Autodesk Inventor part; units mm, degrees
ref_plane "YZ Plane" through (0, 0, 0) normal (1, 0, 0) x (0, 1, 0)
ref_plane "XZ Plane" through (0, 0, 0) normal (0, 1, 0) x (-1, 0, 0)
ref_plane "XY Plane" through (0, 0, 0) normal (0, 0, 1) x (1, 0, 0)
sketch "Sketch1" plane through (0, 0, 0) normal (0, 1, 0) x (-1, 0, 0)
  circle A0 centre (16.272, 0) radius 2.1
  line L0 (14.741, 3.5) -> (19.6914, 3.5)
  line L1 (14.741, -3.5) -> (19.6914, -3.5)
  line L2 (14.741, 3.5) -> (12, 3.5)
  line L3 (14.741, -3.5) -> (12, -3.5)
  line L4 (-2.9689, 12.1423) -> (-6.8146, 18.8032)
  line L5 (-12.8768, 15.3032) -> (-9.0311, 8.6423)
  line L6 (12, -3.5) -> (19.6914, -3.5)
  line L7 (12, 3.5) -> (19.6914, 3.5)
  line L8 (-2.9689, -12.1423) -> (-6.8146, -18.8032)
  line L9 (-9.0311, -8.6423) -> (-12.8768, -15.3032)
  arc A1 (-6.8146, 18.8032) -> (-12.8768, 15.3032) centre (0, 0) ccw
  arc A2 (-12.8768, -15.3032) -> (-6.8146, -18.8032) centre (0, 0) ccw
  arc A3 (19.6914, -3.5) -> (19.6914, 3.5) centre (0, 0) ccw
  arc A4 (-9.0311, 8.6423) -> (-9.0311, -8.6423) centre (0, 0) ccw
  arc A5 (-2.9689, -12.1423) -> (12, -3.5) centre (0, 0) ccw
  arc A6 (12, 3.5) -> (-2.9689, 12.1423) centre (0, 0) ccw
  line L10 (0, 0) -> (16.272, 0)
  circle A7 centre (-8.136, 14.092) radius 2.1
  circle A8 centre (-8.136, -14.092) radius 2.1
  dimension "d6" = 4.2
  dimension "d20" = 16.272
  dimension "d23" = 360
extrude "Extrusion1" add sketch "Sketch1" along normal blind 4
sketch "Sketch2" plane through (0, 4, 0) normal (0, 1, 0) x (1, 0, 0)
  circle A0 centre (0, 0) radius 7.5
extrude "Extrusion2" add sketch "Sketch2" along normal blind 5
sketch "Sketch3" plane through (0, 9, 0) normal (0, 1, 0) x (1, 0, 0)
  circle A0 centre (-4.5, 0) radius 1.35
  circle A1 centre (0, -4.5) radius 1.35
  circle A2 centre (4.5, 0) radius 1.35
  circle A3 centre (0, 4.5) radius 1.35
  point P0 (0, 0)
  point P1 (0, 0)
  dimension "d26" = 2.7
  dimension "d30" = 360
extrude "Extrusion3" cut sketch "Sketch3" against normal through all
sketch "Sketch4" plane through (0, 0, 0) normal (0, -1, 0) x (1, 0, 0)
  circle A0 centre (-4.5, 0) radius 1.35
  circle A1 centre (-4.5, 0) radius 2
  circle A2 centre (0, -4.5) radius 2
  circle A3 centre (4.5, 0) radius 2
  circle A4 centre (0, 4.5) radius 2
  point P0 (0, 0)
  point P1 (0, 0)
  dimension "d34" = 4
  dimension "d37" = 360
extrude "Extrusion4" cut sketch "Sketch4" against normal blind 3
properties part number "Planet_Gear_Output"
Source: CAD feature listing. Evaluate the final solid. Frame: model axes, mm. A direction names the side the tool comes from. Give positions to 0.01 mm unless a question says otherwise; leave off trailing zeros. Write each loop counter-clockwise with the first axis right and the second up, starting at its lowest first coordinate (ties: lowest second). Pieces come first, ordered by that corner, then holes. Notation, with made-up numbers: M 10,-12 L 61,-12 A19 ccw 61,22 Z; hole C 59.25,-29 d5. An arc over 180 degrees is marked long. Return JSON: item names as keys, results as strings. Group by question number.
1) Set-up query: faces 1 (the face through (-3.5, 4, -6.9)), 2 (the face through (-16, 2, -3.5)), 3 (the face through (-20, 2, 0)), 4 (the face through (0, 3, -6)). Return all of +Z, -Z, +X, -X, +Y, -Y with unobstructed straight access to the full face (end or side cutting, diameter ignored); none if empty.
2) Cut plane D-D, the plane z = 0. Output: boundary loops of the cut face in (x, y).
3) Pin query (flat end, axial travel): P1, Ø5, axis at x = 4.5, z = 0, coming from the +Y side; P2, Ø2.5, axis at x = 0, z = 4.5, coming from the -Y side; P3, Ø12, axis at x = -13.5, z = -12.5, coming from the +Y side; P4, Ø4.5, axis at x = -15.5, y = 3, coming from the -Z side. Return the tip coordinate at first contact, or that it passes through.
4) Material intervals for line 1 along Z through (x, y) = (0, 1.8); line 2 along Z through (x, y) = (0, 4.45), sorted ascending. Write a range as [from, to].
5) Pull-direction query (Z, two-part tool) for faces 5 (the face through (-16, 2, 3.5)), 6 (the face through (7.167, 1.972, 15.955)), 7 (the face through (0, 0, 0)); classes: pulls with the +Z half, pulls with the -Z half, needs draft (parallel to the pull), parting line crosses it, or undercut.
6) Cut plane B-B, the plane z = -4.5. Output: boundary loops of the cut face in (x, y).
7) Cut plane A-A, the plane y = 7.75. Output: boundary loops of the cut face in (x, z), plus the area to 3 significant figures.
8) Cut plane C-C, the plane x = 0. Output: boundary loops of the cut face in (y, z).
Recorded:
{
 "1": {"face 1": "+Y", "face 2": "-Z, -X, +Y, -Y", "face 3": "-X, +Y, -Y", "face 4": "-Y"},
 "2": {"outline": "M -20,0 L -18.37,0 L -18.37,4 L -20,4 Z; M -14.17,0 L -6.5,0 L -6.5,3 L -5.85,3 L -5.85,9 L -7.5,9 L -7.5,4 L -14.17,4 Z; M -3.15,3 L -2.5,3 L -2.5,0 L 2.5,0 L 2.5,3 L 3.15,3 L 3.15,9 L -3.15,9 Z; M 5.85,3 L 6.5,3 L 6.5,0 L 12.5,0 L 12.5,4 L 7.5,4 L 7.5,9 L 5.85,9 Z"},
 "3": {"P1": "stops at y = 9", "P2": "passes through", "P3": "stops at y = 4", "P4": "stops at z = -3.5"},
 "4": {"line 1": "z = [-12.5, -6.5], [-2.5, 2.5], [6.5, 12.5]", "line 2": "z = [-7.5, -5.85], [-3.15, 3.15], [5.85, 7.5]"},
 "5": {"face 5": "pulls with the +Z half", "face 6": "undercut", "face 7": "needs draft"},
 "6": {"outline": "M -11.66,0 L -2,0 L -2,3 L -1.35,3 L -1.35,9 L -6,9 L -6,4 L -11.66,4 Z; M 1.35,3 L 2,3 L 2,0 L 11.66,0 L 11.66,4 L 6,4 L 6,9 L 1.35,9 Z"},
 "7": {"outline": "C 0,0 d15; hole C -4.5,0 d2.7; hole C 0,-4.5 d2.7; hole C 0,4.5 d2.7; hole C 4.5,0 d2.7", "area": "154 mm²"},
 "8": {"outline": "M 0,-12.5 L 4,-12.5 L 4,-7.5 L 9,-7.5 L 9,-5.85 L 3,-5.85 L 3,-6.5 L 0,-6.5 Z; M 0,-2.5 L 3,-2.5 L 3,-3.15 L 9,-3.15 L 9,3.15 L 3,3.15 L 3,2.5 L 0,2.5 Z; M 0,6.5 L 3,6.5 L 3,5.85 L 9,5.85 L 9,7.5 L 4,7.5 L 4,12.5 L 0,12.5 Z"}
}
